The listing builds one solid part. Answer for the finished solid, in the listing's coordinates (mm). Coordinates: 2 decimals unless noted, no trailing zeros. Loops run counter-clockwise (first coordinate to the right, second up) from the corner with the lowest first, then second, coordinate; pieces in that order, holes last. Notation, with made-up numbers: (28, 70) - (48, 70) arc R35 cw to (48, 102) - close; hole circle Ø4 at (62, 9.5). An arc over 180 degrees is marked (long way). Put each result on its own line as item: value.
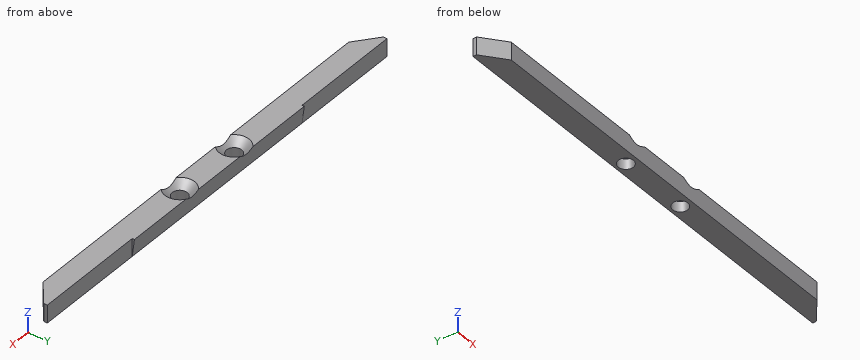
```python
from build123d import *

# Parameters (mm, degrees)
SKETCH_1_W                   = 100
SKETCH_1_H                   = 5.3
EXTRUDE_1_DEPTH              = 4
CUT_EXTRUDE_1_DEPTH          = 101.220207543
SKETCH_3_R                   = 1.5
CUT_EXTRUDE_2_DEPTH          = 101.220207543
HOLE_WIZARD_M3_1_D           = 3.4
HOLE_WIZARD_M3_1_CSINK_D     = 6.72
HOLE_WIZARD_M3_1_CSINK_ANGLE = 90
CUT_EXTRUDE_3_DEPTH          = 101.220207543
CUT_EXTRUDE_4_DEPTH          = 25
CUT_EXTRUDE_5_DEPTH          = 25


with BuildPart() as part:
    # 草图1 → 凸台-拉伸1 (new body)
    with BuildSketch(Plane.XY):
        with Locations((50, 2.65)):
            Rectangle(SKETCH_1_W, SKETCH_1_H)
    extrude(amount=EXTRUDE_1_DEPTH)

    # 草图2 → 切除-拉伸1 (cut, through all)
    with BuildSketch(Plane(origin=(100, 0, 0), x_dir=(0, 0, -1), z_dir=(1, 0, 0))):
        Polygon((-4, 5.3), (0, 5.3), (0, 4.8), align=None)
    extrude(amount=-CUT_EXTRUDE_1_DEPTH, mode=Mode.SUBTRACT)

    # 草图3 → 切除-拉伸2 (cut, through all)
    with BuildSketch(Plane.XY.offset(4)):
        with Locations((42, 2.5)):
            Circle(SKETCH_3_R)
        with Locations(Location((58, 2.5, 0), (0, 0, 180))):
            Circle(SKETCH_3_R)
    extrude(amount=-CUT_EXTRUDE_2_DEPTH, mode=Mode.SUBTRACT)

    # M3 六角凹锥坑螺钉的锥形沉头孔1 (through all)
    with Locations(Plane(origin=(42, 2.5, 4), x_dir=(1, 0, 0), z_dir=(0, 0, 1))):
        with Locations((0, 0), (16, 0)):
            CounterSinkHole(HOLE_WIZARD_M3_1_D / 2, HOLE_WIZARD_M3_1_CSINK_D / 2, counter_sink_angle=HOLE_WIZARD_M3_1_CSINK_ANGLE)

    # 草图6 → 切除-拉伸3 (cut, through all)
    with BuildSketch(Plane.XY.offset(4)):
        Polygon((0, 4), (5, 0), (0, 0), align=None)
        Polygon((100, 0), (100, 4), (95, 0), align=None)
    extrude(amount=-CUT_EXTRUDE_3_DEPTH, mode=Mode.SUBTRACT)

    # 草图7 → 切除-拉伸4 (cut)
    with BuildSketch(Plane(origin=(100, 0, 0), x_dir=(0, 0, -1), z_dir=(1, 0, 0))):
        Polygon((-4, 5.3), (0, 4.8), (-4, 4.8), align=None)
    extrude(amount=-CUT_EXTRUDE_4_DEPTH, mode=Mode.SUBTRACT)

    # 草图8 → 切除-拉伸5 (cut)
    with BuildSketch(Plane.ZY):
        Polygon((0, 4.8), (4, 4.8), (4, 5.3), align=None)
    extrude(amount=-CUT_EXTRUDE_5_DEPTH, mode=Mode.SUBTRACT)


solid = part.part
```
1) The part is cut by section C-C (y = 2.5). Give the vertices of the cut face in (x, z) (3 decimals), and give its area (3 significant figures).
Found:
outline: (1.875, 0) - (40.3, 0) - (40.3, 2.34) - (38.64, 4) - (1.875, 4) - close; (43.7, 0) - (56.3, 0) - (56.3, 2.34) - (54.64, 4) - (45.36, 4) - (43.7, 2.34) - close; (59.7, 0) - (98.125, 0) - (98.125, 4) - (61.36, 4) - (59.7, 2.34) - close
area: 352 mm^2
2) This flat-tipped pin is pushed along its axis until it touches: pin 1 (1 mm diameter, centred on y = 2.5, z = 2, fed in from +X). Where does it stop, or does it pass through?
Found:
pin 1: stops at x = 98.75
3) Straight lines are drawn through the part: L1, parallel to Y at x = 58, z = 1.45; L2, parallel to X at y = 2.5, z = 0.6 (3 decimals); L3, parallel to X at y = 4.65, z = 3.45. For each, find the intervals that lie inside material, in ascending order. Write a range as [from, to].
Found:
L1: y = [0, 0.8], [4.2, 4.98]
L2: x = [1.875, 40.3], [43.7, 56.3], [59.7, 98.125]
L3: x = [0, 40.19], [43.81, 56.19], [59.81, 100]
4) The part is cut by section D-D (x = 20). Give the vertices of the cut face in (y, z).
Found:
outline: (0, 0) - (4.8, 0) - (4.8, 4) - (0, 4) - close
5) The part is cut by section B-B (z = 0.95). Give the vertices of the cut face in (x, y).
Found:
outline: (0, 4) - (5, 0) - (95, 0) - (100, 4) - (100, 4.8) - (75, 4.8) - (75, 4.92) - (25, 4.92) - (25, 4.8) - (0, 4.8) - close; hole circle Ø3.4 at (42, 2.5); hole circle Ø3.4 at (58, 2.5)
6) The part is cut by section A-A (x = 42). Give the vertices of the cut face in (y, z).
Found:
outline: (0, 0) - (0.8, 0) - (0.8, 2.34) - (0, 3.14) - close; (4.2, 0) - (4.8, 0) - (5.22, 3.36) - (4.2, 2.34) - close
